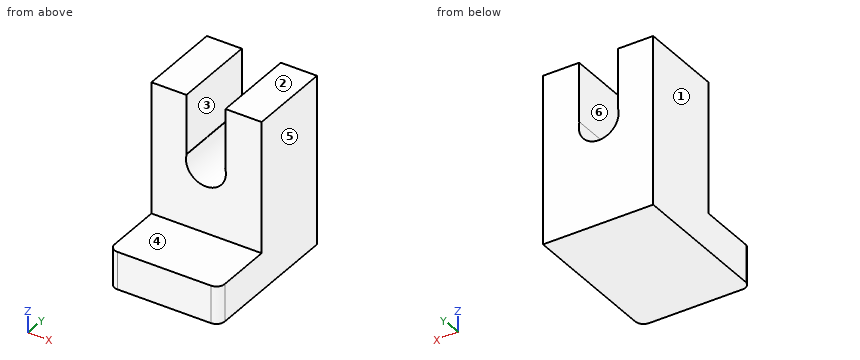
```python
from build123d import *

# Parameters (mm, degrees)
F0_W     = 66.409525
F0_H     = 101.697244
F1_DEPTH = 50.8
F2_W     = 23.525144
F2_H     = 35.777826
F3_DEPTH = 78.232
F4_R     = 12.030111
F5_DEPTH = 92.202
F6_W     = 66.409525
F6_H     = 38.883481
F7_DEPTH = 22.606
F8_R     = 5.08


with BuildPart() as f1:
    # F0 (on Front) → F1 (new body)
    with BuildSketch(Plane.XZ):
        with Locations((0.122526, 5.146127)):
            Rectangle(F0_W, F0_H)
    extrude(amount=F1_DEPTH)

    # F2 (on face) → F3 (cut)
    with BuildSketch(Plane(origin=(0, 0, 0), x_dir=(-1, 0, 0), z_dir=(0, 1, 0))):
        with Locations((0.245053, 38.105836)):
            Rectangle(F2_W, F2_H)
    extrude(amount=-F3_DEPTH, mode=Mode.SUBTRACT)

    # F4 (on face) → F5 (cut)
    with BuildSketch(Plane.XZ.offset(50.8)):
        with Locations((-0.245053, 17.031224)):
            Circle(F4_R)
    extrude(amount=-F5_DEPTH, mode=Mode.SUBTRACT)

    # F6 (on face) → F7 (join)
    with BuildSketch(Plane(origin=(0, 0, -45.702495), x_dir=(1, 0, 0), z_dir=(0, 0, -1))):
        with Locations((0.122526, 70.24174)):
            Rectangle(F6_W, F6_H)
    extrude(amount=-F7_DEPTH)

    # F8
    f8_edges = [f1.edges().sort_by_distance(p)[0] for p in [
        (33.327289, -89.683481, -34.399495),
        (-33.082236, -89.683481, -34.399495),
    ]]
    fillet(f8_edges, radius=F8_R)


solid = f1.part
```
Design review of the part built by this model. Coordinates are the model's own, in mm. Face numbers are marked on the shaded views. A direction names the side the tool comes from. Give positions to 0.01 mm unless a question says otherwise; leave off trailing zeros. Write each loop counter-clockwise with the first axis right and the second up, starting at its lowest first coordinate (ties: lowest second). Pieces come first, ordered by that corner, then holes. Notation, with made-up numbers: (10.25, 42) -> (36.25, 42) arc R17 ccw to (36.25, 64) -> close; hole circle Ø6 at (56.5, 28.25). An arc over 180 degrees is marked (long way). Answer in a Markdown table with one row per item.
(1) Clearance check with a flat-ended pin moving along its axis: pin 1 (5 mm diameter, centred on x = -7.5, z = -16, fed in from -Y). State where the tip first meets the part, or that it passes through.
Results:
| item | result |
|---|---|
| pin 1 | y = -50.8 |
(2) For the marked faces 4, 5 and 6, list the 3-axis set-ups (+Z, -Z, +X, -X, +Y, -Y) from which the entire face can be reached by the end or side of a thin tool; tool diameter is ignored.
Results:
| item | result |
|---|---|
| face 4 | +Z, +X, -X, -Y |
| face 5 | +Z, -Z, +X, +Y, -Y |
| face 6 | +Z, +Y, -Y |
(3) Consider section C-C (x = -14). State the section outline as (y, z) points, then the cut area to 3 significant figures.
Results:
| item | result |
|---|---|
| outline | (-89.68, -45.7) -> (0, -45.7) -> (0, 55.99) -> (-50.8, 55.99) -> (-50.8, -23.1) -> (-89.68, -23.1) -> close |
| area | 6,050 mm2 |
(4) Consider section A-A (z = 26.5). State the section outline as (x, y) points.
Results:
| item | result |
|---|---|
| outline | (-33.08, -50.8) -> (-12.01, -50.8) -> (-12.01, 0) -> (-33.08, 0) -> close; (11.52, -50.8) -> (33.33, -50.8) -> (33.33, 0) -> (11.52, 0) -> close |
(5) Consider section D-D (z = -6.5). State the section outline as (x, y) points.
Results:
| item | result |
|---|---|
| outline | (-33.08, -50.8) -> (33.33, -50.8) -> (33.33, 0) -> (-33.08, 0) -> close |
(6) Consider section B-B (y = -39.5). State the section outline as (x, z) points.
Results:
| item | result |
|---|---|
| outline | (-33.08, -45.7) -> (33.33, -45.7) -> (33.33, 55.99) -> (11.52, 55.99) -> (11.52, 20.22) -> (11.36, 20.22) arc R12.03 cw (long way) to (-11.85, 20.22) -> (-12.01, 20.22) -> (-12.01, 55.99) -> (-33.08, 55.99) -> close |
(7) Mouldability with a two-part tool opening along X and no side actions: class the marked faces 1, 2 and 3 as +X half, -X half, draft (parallel to the pull), parting line (faces both ways), or undercut.
Results:
| item | result |
|---|---|
| face 1 | -X half |
| face 2 | draft |
| face 3 | undercut |
(8) To check wall thickness, follow probe 1 along X at (y, z) = (-30.5, 16.5); probe 2 along X at (y, z) = (-19, 34.5); probe 3 along Y at (x, z) = (-9, 6). State the ranges of each line that lie inside material, in increasing order.
Results:
| item | result |
|---|---|
| probe 1 | -33.08 to -12.26, 11.77 to 33.33 |
| probe 2 | -33.08 to -12.01, 11.52 to 33.33 |
| probe 3 | -50.8 to 0 |
